```python
from build123d import *

# Parameters (mm, degrees)
SKIZZE1_W                       = 20
SKIZZE1_H                       = 20
AUFSATZ_LINEAR_AUSTRAGEN1_DEPTH = 1
SKIZZE2_W                       = 1
SKIZZE2_H                       = 1
AUFSATZ_LINEAR_AUSTRAGEN2_DEPTH = 0.306
SCHNITT_LINEAR_AUSTRAGEN1_DEPTH = 10.306
SKIZZE4_R                       = 0.1
SCHNITT_LINEAR_AUSTRAGEN2_DEPTH = 0.1


with BuildPart() as part:
    # Skizze1 → Aufsatz-Linear austragen1 (new body)
    with BuildSketch(Plane.XY):
        with Locations((-2.517837541, -1.875)):
            Rectangle(SKIZZE1_W, SKIZZE1_H)
    extrude(amount=AUFSATZ_LINEAR_AUSTRAGEN1_DEPTH)

    # Skizze2 → Aufsatz-Linear austragen2 (add)
    with BuildSketch(Plane.XY.offset(1)):
        with Locations((-2.517837541, -1.875)):
            Rectangle(SKIZZE2_W, SKIZZE2_H)
    extrude(amount=AUFSATZ_LINEAR_AUSTRAGEN2_DEPTH)

    # Skizze3 → Schnitt-Linear austragen1 (cut)
    with BuildSketch(Plane.ZY.offset(3.017837541)):
        Polygon((1, -1.375), (1.306, -2.375), (1.306, -1.375), align=None)
    extrude(amount=-SCHNITT_LINEAR_AUSTRAGEN1_DEPTH, mode=Mode.SUBTRACT)

    # Skizze4 → Schnitt-Linear austragen2 (cut)
    with BuildSketch(Plane(origin=(0, 0.162074493, 0.529655205), x_dir=(1, 0, 0), z_dir=(1.0151852031872135e-15, 0.2926072129783145, 0.9562327221513931))):
        with Locations(Location((-2.517837541, -2.130312471, 0), (0, 0, 270))):
            Circle(SKIZZE4_R)
    extrude(amount=-SCHNITT_LINEAR_AUSTRAGEN2_DEPTH, mode=Mode.SUBTRACT)


solid = part.part
```
Work out the finished part from the listing and answer in its coordinate system (mm). Coordinates: 2 decimals unless noted, no trailing zeros. Loops run counter-clockwise (first coordinate to the right, second up) from the corner with the lowest first, then second, coordinate; pieces in that order, holes last. Notation, with made-up numbers: (37, 39.5) - (94, 39.5) arc R12 ccw to (94, 56.5) - close; hole circle Ø8 at (-34, -13.75). An arc over 180 degrees is marked (long way). Use a Markdown table: item, result.
Item 1: Find section B-B, the plane y = 1.75. Determine the outline of the cut face in (x, z).
Evaluation:
| item | result |
|---|---|
| outline | (-12.52, 0) - (7.48, 0) - (7.48, 1) - (-12.52, 1) - close |
Item 2: Given pin 1 Ø3 at (x, y) = (-8.5, -6) entering from -Z; pin 2 Ø10 at (x, y) = (5, 1.5) entering from +Z, each flat-ended and moving along its own axis, determine where each tip first touches the part or whether it passes through.
Evaluation:
| item | result |
|---|---|
| pin 1 | stops at z = 0 |
| pin 2 | stops at z = 1 |
Item 3: Consider probe 1 along Z at (x, y) = (-2, -5.5). Determine where the line is inside the solid, lowest interval first. Write a range as from..to.
Evaluation:
| item | result |
|---|---|
| probe 1 | z = 0..1 |
Item 4: Find section A-A, the plane x = 0. Determine the outline of the cut face in (y, z) (3 decimals).
Evaluation:
| item | result |
|---|---|
| outline | (-11.875, 0) - (8.125, 0) - (8.125, 1) - (-11.875, 1) - close |
